The listing builds one solid part. Answer for the finished solid, in the listing's coordinates (mm). Give positions to 0.01 mm unless a question says otherwise; leave off trailing zeros. Loops run counter-clockwise (first coordinate to the right, second up) from the corner with the lowest first, then second, coordinate; pieces in that order, holes last.
Item 1: Section C-C, the plane y = -0.85 is taken. Give the vertices of the cut face in (x, z).
Item 2: Section A-A, the plane z = 8.75 is taken. Give the vertices of the cut face in (x, y).
Item 3: Each of these flat-tipped pins is pushed along its axis until it touches: pin 1 Ø1 at (x, z) = (1, 15.5) entering from +Y; pin 2 Ø3 at (x, y) = (-1.5, 0.5) entering from -Z; pin 3 Ø1.5 at (y, z) = (1.5, 16.5) entering from +X; pin 4 Ø2 at (y, z) = (-1.5, 6) entering from -X. Where does it stop, or does it pass through?
Item 4: Section B-B, the plane x = -1.35 is taken. Give the vertices of the cut face in (y, z), and give its area (3 significant figures).
Item 5: Section D-D, the plane x = 1.27 is taken. Give the vertices of the cut face in (y, z).
Item 6: Consider line 1 along Z through (x, y) = (1.5, -0.7); line 2 along Y through (x, z) = (0.7, 4.75); line 3 along Y through (x, z) = (1.7, 2.5). Determine where each line is inside the solid, lowest interval first.
from build123d import *

# Parameters (mm, degrees)
SKETCH_1_R      = 2.5
EXTRUDE_1_DEPTH = 5.4
SKETCH_2_R      = 2.5
EXTRUDE_2_DEPTH = 1
SKETCH_3_R      = 0.25
EXTRUDE_3_DEPTH = 12.7


with BuildPart() as part:
    # 草图1 → 拉伸1 (new body)
    with BuildSketch(Plane.XY):
        with Locations(Location((0, 0, 0), (0, 0, 180))):
            Circle(SKETCH_1_R)
    extrude(amount=EXTRUDE_1_DEPTH)

    # 草图2 → 拉伸2 (add)
    with BuildSketch(Plane.XY.offset(5.4)):
        with Locations(Location((0, 0, 0), (0, 0, 180))):
            Circle(SKETCH_2_R)
    extrude(amount=EXTRUDE_2_DEPTH)

    # 草图3 → 拉伸3 (add)
    with BuildSketch(Plane.XY.offset(6.4)):
        with Locations((-1.27, 0)):
            Circle(SKETCH_3_R)
        with Locations(Location((1.27, 0, 0), (0, 0, 180))):
            Circle(SKETCH_3_R)
    extrude(amount=EXTRUDE_3_DEPTH)


solid = part.part
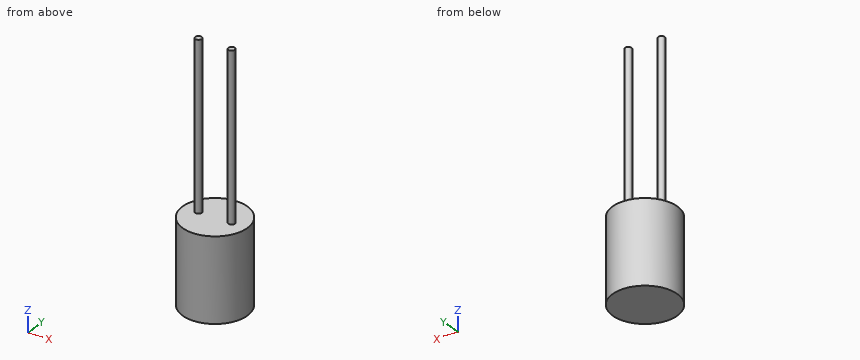
Worked answers:
1. outline: (-2.35, 0) - (2.35, 0) - (2.35, 6.4) - (-2.35, 6.4) - close
2. outline: circle Ø0.5 at (-1.27, 0); circle Ø0.5 at (1.27, 0)
3. pin 1: stops at y = 0.25
3. pin 2: stops at z = 0
3. pin 3: passes through
3. pin 4: stops at x = -2.45
4. outline: (-2.1, 0) - (2.1, 0) - (2.1, 6.4) - (0.24, 6.4) - (0.24, 19.1) - (-0.24, 19.1) - (-0.24, 6.4) - (-2.1, 6.4) - close
4. area: 32.9 mm2
5. outline: (-2.15, 0) - (2.15, 0) - (2.15, 6.4) - (0.25, 6.4) - (0.25, 19.1) - (-0.25, 19.1) - (-0.25, 6.4) - (-2.15, 6.4) - close
6. line 1: z = 0 to 6.4
6. line 2: y = -2.4 to 2.4
6. line 3: y = -1.83 to 1.83
